from build123d import *

# Parameters (mm, degrees)
BOSS_EXTRUDE1_DEPTH = 3.175
BOSS_EXTRUDE2_DEPTH = 6.35
BOSS_EXTRUDE4_DEPTH = 6.35


with BuildPart() as part:
    # Sketch1 → Boss-Extrude1 (new, symmetric)
    with BuildSketch(Plane.XY):
        Polygon((-139.443807584, -165.884900532), (138.870288723, -165.311381671), (121.483295342, -147.92438829), (-121.483295342, -147.92438829), align=None)
    extrude(amount=BOSS_EXTRUDE1_DEPTH, both=True)

    # Sketch2 → Boss-Extrude2 (add)
    with BuildSketch(Plane(origin=(0, 0, -3.175), x_dir=(-1, 0, 0), z_dir=(0, 0, -1))):
        Polygon((-125.686663972, -152.12775692), (-134.666920093, -143.147500799), (-143.647176214, -152.12775692), (-134.666920093, -161.108013041), (-138.870288723, -165.311381671), (139.443807584, -165.884900532), (121.483295342, -147.92438829), (-121.483295342, -147.92438829), align=None)
    extrude(amount=-BOSS_EXTRUDE2_DEPTH)

    # Sketch3 → Boss-Extrude4 (add)
    with BuildSketch(Plane(origin=(0, 0, -3.175), x_dir=(-1, 0, 0), z_dir=(0, 0, -1))):
        Polygon((125.973423403, -152.41451635), (134.953679524, -143.434260229), (143.933935645, -152.41451635), (134.953679524, -161.394772471), align=None)
    extrude(amount=-BOSS_EXTRUDE4_DEPTH)


solid = part.part
Check sheet for the modelled part. Datum: model origin and axes. Units: mm. A direction names the side the tool comes from. Give positions to 0.01 mm unless a question says otherwise; leave off trailing zeros. Order: outer loops, then holes, each group sorted by start corner. A loop starts at its lowest first (then second) coordinate and runs counter-clockwise, first axis right, second up. Notation, with made-up numbers: M 0,-11 L 53,-11 A14 ccw 53,10 Z; hole C 29,-13.75 d11. An arc over 180 degrees is marked long. Answer as CSV lines item,"result". Start each with the question number.
Item 1: Thickness scan on line 1 (X direction, y = -149, z = 2.5); line 2 (X direction, y = -148.5, z = 0.5); line 3 (X direction, y = -145.75, z = -2). Record the ranges inside material, lowest first. Write a range as [from, to].
Item 2: Cross-section at A-A on z = -2. Enter the section's corners in (x, y).
Item 3: Mould release check, pull along Y, two halves, no side actions. Record for faces 1 (the face through (2, -157, 3.175)), 2 (the face through (139.09, -147.57, -0.04)), 3 (the face through (139.22, -156.555, -0.044)): +Y half, -Y half, draft (parallel to the pull), parting line (faces both ways), or undercut.
Item 4: Tool access check on faces 4 (the face through (2, -157, -3.175)), 5 (the face through (-130.4, -147.99, -0.04)), 6 (the face through (-137.17, -163.61, 0.04)). Record the directions out of +Z, -Z, +X, -X, +Y, -Y that give a thin tool (end or side, any length) a straight path to the whole face; none if there is none.
Item 5: Cross-section at B-B on y = -157.75. Enter the section's corners in (x, z) (3 decimals).
Item 6: Cross-section at C-C on x = -54. Enter the section's corners in (y, z) (3 decimals), plus the area to 3 significant figures.
Item 7: Gauge pin test, flat ends, axial feed: P1, Ø1.9, axis at x = -48, z = 0, coming from the +Y side; P2, Ø1.5, axis at y = -156.5, z = 1, coming from the -X side. Record the tip position at first contact, or that the pin passes through.
Established:
1,line 1,"x = [-140.52, -129.39], [-122.56, 122.56], [128.81, 140.52]"
1,line 2,"x = [-140.02, -129.89], [-122.06, 122.06], [129.31, 140.02]"
1,line 3,"x = [-137.27, -132.64], [132.06, 137.27]"
2,outline,"M -143.93,-152.41 L -134.95,-161.39 L -139.44,-165.88 L 138.87,-165.31 L 134.67,-161.11 L 143.65,-152.13 L 134.67,-143.15 L 125.69,-152.13 L 121.48,-147.92 L -121.48,-147.92 L -125.97,-152.41 L -134.95,-143.43 Z"
3,face 1,"draft"
3,face 2,"+Y half"
3,face 3,"undercut"
4,face 4,"-Z, +X, -X, +Y, -Y"
4,face 5,"+Z, -Z, +Y"
4,face 6,"+Z, -Z, -X"
5,outline,"M -138.598,-3.175 L 138.025,-3.175 L 138.025,3.175 L -138.598,3.175 Z"
6,outline,"M -165.709,-3.175 L -147.924,-3.175 L -147.924,3.175 L -165.709,3.175 Z"
6,area,"113 mm^2"
7,P1,"stops at y = -147.92"
7,P2,"stops at x = -140.6"
